```python
from build123d import *

# Parameters (mm, degrees)
SKETCH_1_R      = 20
SKETCH_1_R_2    = 6.5
EXTRUDE_1_DEPTH = 70
EXTRUDE_2_DEPTH = 25
SKETCH_2_4_R    = 6.5
EXTRUDE_4_DEPTH = 1
EXTRUDE_START   = -25
SKETCH_3_R      = 5
EXTRUDE_5_DEPTH = 25
SKETCH_4_R      = 6.5
EXTRUDE_6_DEPTH = 13


with BuildPart() as part:
    # Sketch 1 → Extrude 1 (new body)
    with BuildSketch(Plane.XY):
        Circle(SKETCH_1_R)
        Circle(SKETCH_1_R_2, mode=Mode.SUBTRACT)
    extrude(amount=EXTRUDE_1_DEPTH)



with BuildPart() as body_2:
    # Sketch 2 → Extrude 2 (new body)
    with BuildSketch(Plane.XY.offset(70)):
        with BuildLine():
            ThreePointArc((20, 0), (-8.660254038, -18.027756377), (-12.5, 15.612494996))
            Line((-12.5, 15.612494996), (-12.5, 27.271780287))
            ThreePointArc((-12.5, 27.271780287), (-16.201851746, -25.248762346), (30, 0))
            ThreePointArc((30, 0), (25.248762346, 16.201851746), (12.5, 27.271780287))
            Line((12.5, 27.271780287), (12.5, 15.612494996))
            ThreePointArc((12.5, 15.612494996), (18.027756377, 8.660254038), (20, 0))
        make_face()
        with BuildLine():
            Line((-12.5, 27.271780287), (-12.5, 15.612494996))
            ThreePointArc((-12.5, 15.612494996), (-10.106596746, 17.258525494), (-7.5, 18.540496218))
            Line((-7.5, 18.540496218), (-7.5, 29.047375097))
            ThreePointArc((-7.5, 29.047375097), (-10.039331862, 28.270334554), (-12.5, 27.271780287))
        make_face()
        with BuildLine():
            ThreePointArc((7.5, 18.540496218), (10.106596746, 17.258525494), (12.5, 15.612494996))
            Line((12.5, 15.612494996), (12.5, 27.271780287))
            ThreePointArc((12.5, 27.271780287), (10.039331862, 28.270334554), (7.5, 29.047375097))
            Line((7.5, 29.047375097), (7.5, 18.540496218))
        make_face()
        with BuildLine():
            Line((-12.5, 55), (-12.5, 27.271780287))
            ThreePointArc((-12.5, 27.271780287), (-10.039331862, 28.270334554), (-7.5, 29.047375097))
            Line((-7.5, 29.047375097), (-7.5, 55))
            ThreePointArc((-7.5, 55), (0, 62.5), (7.5, 55))
            Line((7.5, 55), (7.5, 29.047375097))
            ThreePointArc((7.5, 29.047375097), (10.039331862, 28.270334554), (12.5, 27.271780287))
            Line((12.5, 27.271780287), (12.5, 55))
            ThreePointArc((12.5, 55), (0, 67.5), (-12.5, 55))
        make_face()
    extrude(amount=EXTRUDE_2_DEPTH)


with BuildPart() as part_1:
    add(part.part)

    add(body_2.part)  # Extrude 4 merges body 2
    # Sketch 2_4 → Extrude 4 (add)
    with BuildSketch(Plane.XY.offset(70)):
        with BuildLine():
            Line((7.5, 18.540496218), (7.5, 55))
            ThreePointArc((7.5, 55), (0, 62.5), (-7.5, 55))
            Line((-7.5, 55), (-7.5, 18.540496218))
            ThreePointArc((-7.5, 18.540496218), (0, -20), (7.5, 18.540496218))
        make_face()
        Circle(SKETCH_2_4_R, mode=Mode.SUBTRACT)
    extrude(amount=EXTRUDE_4_DEPTH)

    # Sketch 3 → Extrude 5 (add)
    with BuildSketch(Plane.XY.offset(95).offset(EXTRUDE_START)):
        with BuildLine():
            Line((28.660254038, -29.641016151), (22.802389662, -19.494897428))
            ThreePointArc((22.802389662, -19.494897428), (15, -25.980762114), (5.481881586, -29.494897428))
            Line((5.481881586, -29.494897428), (11.339745962, -39.641016151))
            ThreePointArc((11.339745962, -39.641016151), (25, -43.301270189), (28.660254038, -29.641016151))
        make_face()
        with Locations((20, -34.641016151)):
            Circle(SKETCH_3_R, mode=Mode.SUBTRACT)
    extrude(amount=EXTRUDE_5_DEPTH)

    # Sketch 4 → Extrude 6 (add)
    with BuildSketch(Plane.XY.offset(71)):
        with BuildLine():
            Line((7.5, 18.540496218), (7.5, 55))
            ThreePointArc((7.5, 55), (0, 62.5), (-7.5, 55))
            Line((-7.5, 55), (-7.5, 18.540496218))
            ThreePointArc((-7.5, 18.540496218), (0, -20), (7.5, 18.540496218))
        make_face()
        Circle(SKETCH_4_R, mode=Mode.SUBTRACT)
    extrude(amount=EXTRUDE_6_DEPTH)


solid = part_1.part
```
Source: CAD feature listing. Evaluate the final solid. Frame: model axes, mm. A direction names the side the tool comes from. Round coordinates to 2 decimals unless told otherwise and drop trailing zeros. Loops run counter-clockwise (first coordinate to the right, second up) from the corner with the lowest first, then second, coordinate; pieces in that order, holes last. Notation, with made-up numbers: (29.5, 38) - (55.5, 38) arc R27 cw to (55.5, 55) - close; hole circle Ø11 at (87, 30.5). An arc over 180 degrees is marked (long way). Use CSV: the item, a comma, the result in double quotes.
Q1. Section query A-A, the plane x = 0. Output: boundary loops of the cut face in (y, z).
Reported:
outline,"(-30, 70) - (-20, 70) - (-20, 0) - (-6.5, 0) - (-6.5, 84) - (-20, 84) - (-20, 95) - (-30, 95) - close; (6.5, 0) - (20, 0) - (20, 70) - (67.5, 70) - (67.5, 95) - (62.5, 95) - (62.5, 84) - (6.5, 84) - close"
Q2. Section query B-B, the plane z = 76. Output: boundary loops of the cut face in (x, y), then the cut area to 3 significant figures.
Reported:
outline,"(-12.5, 27.27) arc R30 ccw to (5.48, -29.49) - (11.34, -39.64) arc R10 ccw to (28.66, -29.64) - (22.8, -19.49) arc R30 ccw to (12.5, 27.27) - (12.5, 55) arc R12.5 ccw to (-12.5, 55) - close; hole circle Ø13 at (0, 0); hole circle Ø10 at (20, -34.64)"
area,"3,880 mm^2"
Q3. Ray query, line 1 along Y through (x, z) = (0, 89); line 2 along X through (y, z) = (0, 86.5); line 3 along Y through (x, z) = (-0.5, 5.5). Return the intervals inside material, ascending.
Reported:
line 1,"-30 to -20, 62.5 to 67.5"
line 2,"-30 to -20, 20 to 30"
line 3,"-19.99 to -6.48, 6.48 to 19.99"
Q4. Mould query, pull axis Y, two halves, no side actions, for faces 4 (the cylindrical face through (-28.777, -8.478, 82.325)), 5 (the flat face through (18, 12, 95)), 6 (the cylindrical face through (19.349, -29.684, 82.325)), 7 (the flat face through (-7.5, 37, 89)). Classes: pulls with the +Y half, pulls with the -Y half, needs draft (parallel to the pull), parting line crosses it, or undercut.
Reported:
face 4,"parting line crosses it"
face 5,"needs draft"
face 6,"undercut"
face 7,"undercut"
Q5. Pin query (flat end, axial travel): pin 1 Ø4 at (x, z) = (8, 44) entering from +Y; pin 2 Ø12.5 at (y, z) = (46, 79) entering from +X; pin 3 Ø10.5 at (x, y) = (0, 0) entering from +Z; pin 4 Ø12 at (y, z) = (37, 87) entering from -X. Return the tip coordinate at first contact, or that it passes through.
Reported:
pin 1,"y = 19.08"
pin 2,"x = 12.5"
pin 3,"through"
pin 4,"x = -12.5"
Q6. Reachability of faces 1 (the flat face through (7.5, 37, 89)), 2 (the flat face through (-12.5, 41, 82)), 3 (the flat face through (25.772, -24.639, 82.325)) from +Z, -Z, +X, -X, +Y, -Y: full face, straight path, thin tool, end or side. Return the list, or none.
Reported:
face 1,"+Z"
face 2,"+Z, -Z, -X, +Y"
face 3,"+Z, -Z, +X"
Q7. Section query C-C, the plane y = 44. Output: boundary loops of the cut face in (x, z), then the cut area to 3 significant figures.
Reported:
outline,"(-12.5, 70) - (12.5, 70) - (12.5, 95) - (7.5, 95) - (7.5, 84) - (-7.5, 84) - (-7.5, 95) - (-12.5, 95) - close"
area,"460 mm^2"
Q8. Section query D-D, the plane x = 17. Output: boundary loops of the cut face in (y, z), then the cut area to 3 significant figures.
Reported:
outline,"(-44.18, 70) - (-38.64, 70) - (-38.64, 95) - (-44.18, 95) - close; (-30.64, 70) - (-10.54, 70) - (-10.54, 0) - (10.54, 0) - (10.54, 70) - (24.72, 70) - (24.72, 95) - (10.54, 95) - (10.54, 84) - (-10.54, 84) - (-10.54, 95) - (-30.64, 95) - close"
area,"2,770 mm^2"
